Autodesk Inventor part; units mm, degrees
ref_plane "YZ Plane" through (0, 0, 0) normal (1, 0, 0) x (0, 1, 0)
ref_plane "XZ Plane" through (0, 0, 0) normal (0, 1, 0) x (-1, 0, 0)
ref_plane "XY Plane" through (0, 0, 0) normal (0, 0, 1) x (1, 0, 0)
sketch "Sketch1" plane through (0, 0, 0) normal (0, 0, 1) x (1, 0, 0)
  line L0 (0, 0) -> (69.215, 0)
  line L1 (69.215, 0) -> (69.215, -254)
  line L2 (69.215, -254) -> (0, -254)
  line L3 (0, -254) -> (0, 0)
  dimension "d0" = 69.215
  dimension "d1" = 254
extrude "Extrusion1" add sketch "Sketch1" along normal blind 9.525
sketch "Sketch4" plane through (0, 0, 0) normal (0, 0, -1) x (-1, 0, 0)
  line L0 (-69.215, -254) -> (0, -254)
  line L1 (0, 0) -> (-24.765, 0)
  line L2 (-24.765, 0) -> (-24.765, -254)
  line L3 (-24.765, -254) -> (0, -254)
  line L4 (0, -254) -> (0, 0)
  dimension "d11" = 24.765
extrude "Extrusion4" cut sketch "Sketch4" against normal blind 127
sketch "Sketch5" plane through (69.215, -254, 0) normal (0, -1, 0) x (1, 0, 0)
  point P0 (-69.215, 0)
sketch "Sketch9" plane through (69.215, -254, 0) normal (0, -1, 0) x (1, 0, 0)
  line L0 (-44.45, 9.525) -> (-44.45, 0)
  line L1 (0, 0) -> (0, 9.525)
  point P0 (-69.215, 0)
  point P1 (-12.7, 4.7625)
  point P2 (-31.75, 4.7625)
hole "Hole2" at (37.465, -254, 4.7625) at (56.515, -254, 4.7625) direction (0, 1, 0) diameter 3.302 depth 7.62 tip angle 118
sketch "Sketch11" plane through (69.215, 0, 9.525) normal (0, 1, 0) x (1, 0, 0)
  line L0 (-38.1, -46.0375) -> (-44.45, -46.0375)
  line L1 (-44.45, -46.0375) -> (-44.45, 55.5625)
  line L2 (-44.45, 55.5625) -> (-38.1, 55.5625)
  line L3 (-38.1, 55.5625) -> (-38.1, -46.0375)
  line L4 (-44.45, 9.525) -> (-44.45, 0)
  line L5 (0, 0) -> (-44.45, 0)
  line L6 (0, 9.525) -> (0, 0)
  line L7 (-44.45, 9.525) -> (0, 9.525)
  point P0 (-69.215, 9.525)
  dimension "d41" = 6.35
  dimension "d42" = 101.6
  dimension "d44" = 9.525
  dimension "d45" = 46.0375
  dimension "d46" = 0
extrude "Extrusion7" add sketch "Sketch11" along normal blind 12.7 contours L0 L1 L5 L3 | L5 L1 L7 L3 | L7 L1 L2 L3
sketch "Sketch12" plane through (24.765, -254, 0) normal (-1, 0, 0) x (0, 0, 1)
  line L0 (9.525, 254) -> (9.525, 0)
  line L1 (55.5625, 254) -> (9.525, 254)
  line L2 (55.5625, 254) -> (55.5625, 266.7)
  line L3 (-46.0375, 266.7) -> (55.5625, 266.7)
  line L4 (-46.0375, 254) -> (-46.0375, 266.7)
  line L5 (0, 254) -> (-46.0375, 254)
  line L6 (0, 0) -> (0, 254)
  line L7 (9.525, 0) -> (0, 0)
  point P0 (-39.6875, 260.35)
  point P1 (49.2125, 260.35)
  dimension "d49" = 12.7
  dimension "d50" = 6.35
  dimension "d51" = 6.35
  dimension "d52" = 6.35
  dimension "d53" = 6.35
hole "Hole3" at (24.765, 6.35, -39.6875) at (24.765, 6.35, 49.2125) direction (1, 0, 0) diameter 6.35 depth 25.4 tip angle 118
equation "\"d45\" = -0.5 * d44 + 0.5 * d42"
properties part number "LeftSideTopPlateConnector"
Work out the finished part from the listing and answer in its coordinate system (mm). A direction names the side the tool comes from. Round coordinates to 2 decimals unless told otherwise and drop trailing zeros. Write each loop counter-clockwise with the first axis right and the second up, starting at its lowest first coordinate (ties: lowest second). Pieces come first, ordered by that corner, then holes. Notation, with made-up numbers: (72, 78.25) -> (77, 78.25) arc R35 ccw to (77, 113.25) -> close; hole circle Ø7 at (79.5, -15.75). An arc over 180 degrees is marked (long way). Answer as CSV lines item,"result". Start each with the question number.
(1) The mould has two halves that part along Y. Classify faces 4 (the flat face through (28, 0, 32)), 5 (the cylindrical face through (27.98, 9.45, 48.52)), 6 (the flat face through (31.115, 6, 4)): +Y half, -Y half, draft (parallel to the pull), parting line (faces both ways), or undercut.
(2) The part is cut by section B-B, the plane z = -2.5. Give the vertices of the cut face in (x, y) (3 decimals).
(3) The part is cut by section C-C, the plane x = 49. Give the vertices of the cut face in (y, z) (3 decimals).
(4) A tool of negligible diameter and unlimited length cuts with its end or side. For faces 1 (the flat face through (28, 0, -23)), 2 (the flat face through (28, 12.7, 4)), 3 (the flat face through (50, 0, 5)), from which of +Z, -Z, +X, -X, +Y, -Y can it reach the whole face along a straight path? Write none if from no direction.
(5) The part is cut by section A-A, the plane y = 6.35. Give the vertices of the cut face in (x, z) (1 decimal), then the cut area to 3 significant figures.
(6) Find the intervals of material crossed by probe 1 along Z at (x, y) = (29, 6); probe 2 along Z at (x, y) = (67, -207) (3 decimals); probe 3 along Y at (x, z) = (30.5, 34.5), in increasing order.
(7) Each of these flat-tipped pins is pushed along its axis until it touches: pin 1 (5 mm diameter, centred on x = 30.5, z = 35, fed in from -Y); pin 2 (4 mm diameter, centred on x = 31, y = -157, fed in from -Z); pin 3 (4 mm diameter, centred on x = 36, y = -192.5, fed in from +Z) (3 decimals); pin 4 (3 mm diameter, centred on y = -104, z = 10.5, fed in from -X) (3 decimals). Where does it stop, or does it pass through?
Output values:
1,face 4,"-Y half"
1,face 5,"undercut"
1,face 6,"draft"
2,outline,"(24.765, 0) -> (31.115, 0) -> (31.115, 12.7) -> (24.765, 12.7) -> close"
3,outline,"(-254, 0) -> (0, 0) -> (0, 9.525) -> (-254, 9.525) -> close"
4,face 1,"-Z, +X, -X, -Y"
4,face 2,"+Z, -Z, +X, -X, +Y"
4,face 3,"+Z, -Z, +X, +Y"
5,outline,"(24.8, -46) -> (31.1, -46) -> (31.1, -42.9) -> (24.8, -42.9) -> close; (24.8, -36.5) -> (31.1, -36.5) -> (31.1, 46) -> (24.8, 46) -> close; (24.8, 52.4) -> (31.1, 52.4) -> (31.1, 55.6) -> (24.8, 55.6) -> close"
5,area,"565 mm²"
6,probe 1,"z = -46.04 to -42.84, -36.53 to 46.06, 52.37 to 55.56"
6,probe 2,"z = 0 to 9.525"
6,probe 3,"y = 0 to 12.7"
7,pin 1,"stops at y = 0"
7,pin 2,"stops at z = 0"
7,pin 3,"stops at z = 9.525"
7,pin 4,"stops at x = 24.765"
